Input: part model. Units: mm. Frame: model coordinates. A direction names the side the tool comes from. Give positions to 0.01 mm unless a question says otherwise; leave off trailing zeros. Write each loop counter-clockwise with the first axis right and the second up, starting at its lowest first coordinate (ties: lowest second). Pieces come first, ordered by that corner, then holes. Notation, with made-up numbers: (-0.75, 16.25) - (52.25, 16.25) arc R20 ccw to (52.25, 52.25) - close; hole circle Ø6 at (39, 68.25). An arc over 180 degrees is marked (long way). Answer as a JSON object with one key per item and string values. Group by question number.
from build123d import *

# Parameters (mm, degrees)
F0_W     = 60
F0_H     = 23
F1_DEPTH = 30
F2_R     = 5
F3_R     = 2
F4_DEPTH = 13


with BuildPart() as f1:
    # F0 (on Top) → F1 (new body)
    with BuildSketch(Plane.XY):
        Rectangle(F0_W, F0_H)
    extrude(amount=F1_DEPTH)

    # F2
    f2_edges = [f1.edges().sort_by_distance(p)[0] for p in [
        (-30, 11.5, 15),
        (-30, -11.5, 15),
        (30, -11.5, 15),
        (30, 11.5, 15),
        (0, -11.5, 30),
        (-30, 0, 30),
        (0, 11.5, 30),
        (30, 0, 30),
    ]]
    fillet(f2_edges, radius=F2_R)

    # F3 (on Front) → F4 (join)
    with BuildSketch(Plane.XZ):
        with Locations((-15, 9.963796)):
            Circle(F3_R)
        with BuildLine():
            ThreePointArc((17, 9.963796), (15, 11.963796), (13, 9.963796))
            ThreePointArc((13, 9.963796), (15, 7.963796), (17, 9.963796))
        make_face()
        with BuildLine():
            ThreePointArc((7, 9.963796), (5, 11.963796), (3, 9.963796))
            Line((3, 9.963796), (7, 9.963796))
        make_face()
        with BuildLine():
            Line((7, 9.963796), (3, 9.963796))
            ThreePointArc((3, 9.963796), (5, 7.963796), (7, 9.963796))
        make_face()
        with BuildLine():
            ThreePointArc((-3, 9.963796), (-5, 11.963796), (-7, 9.963796))
            Line((-7, 9.963796), (-3, 9.963796))
        make_face()
        with BuildLine():
            Line((-3, 9.963796), (-7, 9.963796))
            ThreePointArc((-7, 9.963796), (-5, 7.963796), (-3, 9.963796))
        make_face()
    extrude(amount=F4_DEPTH)


solid = f1.part
1) Mould query, pull axis X, two halves, no side actions, for faces 1 (the face through (30, 0, 12)), 2 (the face through (0.35, -10.07, 28.5)), 3 (the face through (15.26, -12.24, 7.98)), 4 (the face through (5.26, -12.24, 7.98)). Classes: +X half, -X half, draft (parallel to the pull), parting line (faces both ways), or undercut.
2) Line query: line 1 along Y through (x, z) = (5, 20); line 2 along X through (y, z) = (8, 12.75); line 3 along Z through (x, y) = (-15.5, -9.5). Output: solid intervals per line, ascending. Write a range as from..to.
3) Cut plane A-A on x = -15. Return the cut outline in (y, z), and give its area (3 significant figures).
4) Cut plane B-B on z = 2. Return the cut outline in (x, y), and give its area (3 significant figures).
5) Cut plane C-C on y = 10.25. Return the cut outline in (x, z), and give its area (3 significant figures).
6) Reachability of faces 5 (the face through (-3.53, -12.24, 8.61)), 6 (the face through (-30, 0, 12)) from +Z, -Z, +X, -X, +Y, -Y: full face, straight path, thin tool, end or side. Return the list, or none.
7) Pin query (flat end, axial travel): P1, Ø6, axis at x = -21.5, z = 20, coming from the -Y side; P2, Ø1, axis at y = -9, z = 26.5, coming from the +X side. Return the tip coordinate at first contact, or that it passes through.
8) Cut plane D-D on x = -21. Return the cut outline in (y, z).
Filled in:
{
 "1": {"face 1": "+X half", "face 2": "draft", "face 3": "undercut", "face 4": "undercut"},
 "2": {"line 1": "y = -11.5..11.5", "line 2": "x = -29.77..29.77", "line 3": "z = 0..29"},
 "3": {"outline": "(-13, 7.96) - (-11.5, 7.96) - (-11.5, 0) - (11.5, 0) - (11.5, 25) arc R5 ccw to (6.5, 30) - (-6.5, 30) arc R5 ccw to (-11.5, 25) - (-11.5, 11.96) - (-13, 11.96) - close", "area": "685 mm²"},
 "4": {"outline": "(-30, -6.5) arc R5 ccw to (-25, -11.5) - (25, -11.5) arc R5 ccw to (30, -6.5) - (30, 6.5) arc R5 ccw to (25, 11.5) - (-25, 11.5) arc R5 ccw to (-30, 6.5) - close", "area": "1,360 mm²"},
 "5": {"outline": "(-28.31, 0) - (28.31, 0) - (28.31, 25) arc R3.31 ccw to (25, 28.31) - (-25, 28.31) arc R3.31 ccw to (-28.31, 25) - close", "area": "1,600 mm²"},
 "6": {"face 5": "-Y", "face 6": "+Z, -Z, -X, +Y, -Y"},
 "7": {"P1": "stops at y = -11.5", "P2": "stops at x = 29.38"},
 "8": {"outline": "(-11.5, 0) - (11.5, 0) - (11.5, 25) arc R5 ccw to (6.5, 30) - (-6.5, 30) arc R5 ccw to (-11.5, 25) - close"}
}
